from build123d import *

# Parameters (mm, degrees)
FILLET1_R          = 2
SKETCH4_R          = 10.5
CUT_EXTRUDE3_DEPTH = 6
SKETCH5_R          = 1.25
CUT_EXTRUDE4_DEPTH = 16.75
SKETCH6_R          = 2.5
CUT_EXTRUDE5_DEPTH = 11.75
FILLET2_R          = 3


with BuildPart() as part:
    # Sketch1 → Revolve1 (revolve)
    with BuildSketch(Plane(origin=(0, 0, 0), x_dir=(1, 0, 0), z_dir=(0, 1, 0))):
        Polygon((-4.630434783, 14.4), (7.869565217, 14.4), (10.619565217, 11.390476118), (10.619565217, 4), (14.619565217, 4), (14.619565217, 0), (13.372742768, 0), (-6.130434783, 0), (-6.130434783, 18.2), (-4.630434783, 18.2), align=None)
    revolve(axis=Axis((-12.391304348, 0, 0), (1, 0, 0)))

    # Fillet1
    fillet1_edges = [part.edges().sort_by_distance(p)[0] for p in [
        (14.619565217, 0, 4),
    ]]
    fillet(fillet1_edges, radius=FILLET1_R)

    # Sketch4 → Cut-Extrude3 (cut)
    with BuildSketch(Plane.ZY.offset(6.130434783)):
        Circle(SKETCH4_R)
    extrude(amount=-CUT_EXTRUDE3_DEPTH, mode=Mode.SUBTRACT)

    # Sketch5 → Cut-Extrude4 (cut)
    with BuildSketch(Plane(origin=(10.619565217, 0, 0), x_dir=(0, 0, -1), z_dir=(1, 0, 0))):
        with Locations((0, 9)):
            Circle(SKETCH5_R)
        with Locations((6.363961031, 6.363961031)):
            Circle(SKETCH5_R)
        with Locations((9, 0)):
            Circle(SKETCH5_R)
        with Locations((6.363961031, -6.363961031)):
            Circle(SKETCH5_R)
        with Locations((0, -9)):
            Circle(SKETCH5_R)
        with Locations((-6.363961031, -6.363961031)):
            Circle(SKETCH5_R)
        with Locations((-9, 0)):
            Circle(SKETCH5_R)
        with Locations((-6.363961031, 6.363961031)):
            Circle(SKETCH5_R)
    extrude(amount=-CUT_EXTRUDE4_DEPTH, mode=Mode.SUBTRACT)

    # Sketch6 → Cut-Extrude5 (cut)
    with BuildSketch(Plane.ZY.offset(6.130434783)):
        with Locations((0, 9)):
            Circle(SKETCH6_R)
        with Locations((6.363961031, 6.363961031)):
            Circle(SKETCH6_R)
        with Locations((9, 0)):
            Circle(SKETCH6_R)
        with Locations((6.363961031, -6.363961031)):
            Circle(SKETCH6_R)
        with Locations((0, -9)):
            Circle(SKETCH6_R)
        with Locations((-6.363961031, -6.363961031)):
            Circle(SKETCH6_R)
        with Locations((-9, 0)):
            Circle(SKETCH6_R)
        with Locations((-6.363961031, 6.363961031)):
            Circle(SKETCH6_R)
    extrude(amount=-CUT_EXTRUDE5_DEPTH, mode=Mode.SUBTRACT)

    # Fillet2
    fillet2_edges = [part.edges().sort_by_distance(p)[0] for p in [
        (7.869565217, 0, 14.4),
        (10.619565217, 0, 11.390476118),
    ]]
    fillet(fillet2_edges, radius=FILLET2_R)


solid = part.part
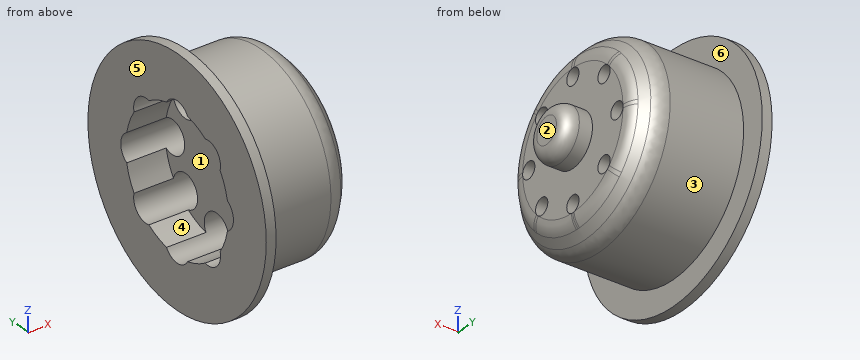
Read the model definition and answer for the solid it produces. Units are mm, in the model's axes. Face numbers are marked on the shaded views. A direction names the side the tool comes from. Round coordinates to 2 decimals unless told otherwise and drop trailing zeros. Order: outer loops, then holes, each group sorted by start corner. A loop starts at its lowest first (then second) coordinate and runs counter-clockwise, first axis right, second up. Notation, with made-up numbers: (-27.75, -16.5) - (4.25, -16.5) arc R14 cw to (4.25, -3.5) - close; hole circle Ø7 at (55, -40). An arc over 180 degrees is marked (long way). Use one line per item in the form item = value. Start each with the question number.
(1) Flat-ended cylindrical pins translate along their axes: pin 1 Ø4 at (y, z) = (6.36, -6.36) entering from -X; pin 2 Ø5 at (x, z) = (11, 12) entering from -Y; pin 3 Ø6 at (y, z) = (6.36, 6.36) entering from +X; pin 4 Ø2 at (y, z) = (0, -9) entering from -X. Find the tip coordinate at first contact, or state that the pin passes through.
(2) Determine the mould class of the marked faces 1, 2 and 3 for opening direction Y: +Y half, -Y half, draft (parallel to the pull), parting line (faces both ways), or undercut.
(3) For the marked faces 4, 5 and 6, determine the directions among +Z, -Z, +X, -X, +Y, -Y from which every point of the face is accessible in a straight line to the end or side of a thin tool.
(4) Find the intervals of material crossed by line 1 along Y through (x, z) = (0.5, -2); line 2 along Y through (x, z) = (5.75, 6); line 3 along Z through (x, y) = (-2.75, 0), in increasing order. Write a range as from..to.
(5) The part is cut by section B-B (x = 3). Count the separate pieces of the cut face and the enclosed holes in it, then the cut area to 3 significant figures.
(6) The part is cut by section A-A (x = -2.5). Give the vertices of the cut face in (y, z), then the cut area to 3 significant figures.
Checked values:
q1.pin_1 = 5.62
q1.pin_2 = -7.94
q1.pin_3 = 10.62
q1.pin_4 = through
q2.face_1 = undercut
q2.face_2 = draft
q2.face_3 = parting line
q3.face_4 = -X
q3.face_5 = +Z, -Z, -X, +Y, -Y
q3.face_6 = +X
q4.line_1 = -14.26..-10.5, -7.5..7.5, 10.5..14.26
q4.line_2 = -13.09..-7.56, -5.17..5.17, 7.56..13.09
q4.line_3 = -14.4..-11.5, 11.5..14.4
q5.separate_pieces = 1
q5.enclosed_holes = 8
q5.area = 494 mm^2
q6.outline = circle Ø28.8 at (0, 0); hole (-10.28, -2.15) arc R10.5 ccw to (-8.79, -5.75) arc R2.5 ccw to (-5.75, -8.79) arc R10.5 ccw to (-2.15, -10.28) arc R2.5 ccw to (2.15, -10.28) arc R10.5 ccw to (5.75, -8.79) arc R2.5 ccw to (8.79, -5.75) arc R10.5 ccw to (10.28, -2.15) arc R2.5 ccw to (10.28, 2.15) arc R10.5 ccw to (8.79, 5.75) arc R2.5 ccw to (5.75, 8.79) arc R10.5 ccw to (2.15, 10.28) arc R2.5 ccw to (-2.15, 10.28) arc R10.5 ccw to (-5.75, 8.79) arc R2.5 ccw to (-8.79, 5.75) arc R10.5 ccw to (-10.28, 2.15) arc R2.5 ccw to start
q6.area = 280 mm^2
